The drawing under review shows one solid part. Ordinate dimensions are in mm from its lowest x, y, z. A direction names the side the tool comes from. Give positions to 0.01 mm unless a question says otherwise; leave off trailing zeros. Write each loop counter-clockwise with the first axis right and the second up, starting at its lowest first coordinate (ties: lowest second). Pieces come first, ordered by that corner, then holes. Notation, with made-up numbers: M -36,-4.75 L 11,-4.75 A28 cw 11,15.25 Z; hole C -13,16 d5. An arc over 180 degrees is marked long. Write each question's results on one line, items separated by ' | '. Start each with the question number.
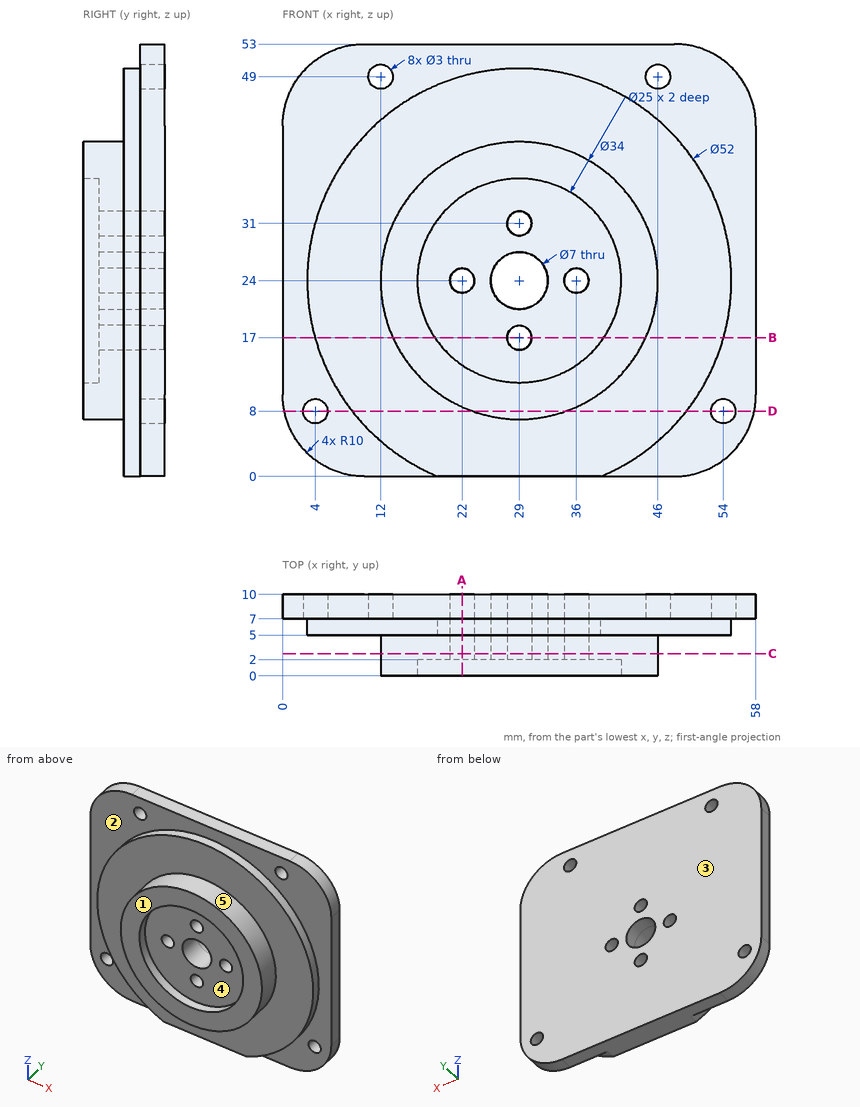
Q1. We need section B-B on z = 17. Write out the cut boundary in (x, y).
Q2. For pin 1 Ø3.5 at (x, z) = (22, 24) entering from -Y; pin 2 Ø2.5 at (x, z) = (22, 24) entering from +Y; pin 3 Ø1.5 at (y, z) = (1, 23) entering from +X; pin 4 Ø1 at (x, y) = (23.5, 1.5) entering from +Z, all flat-tipped, find the tip position at first contact; note any pin that passes through.
Q3. We need section D-D on z = 8. Write out the cut boundary in (x, y).
Q4. Wall thickness on line 1 along X through (y, z) = (5.25, 24); line 2 along X through (y, z) = (4.55, 24); line 3 along X through (y, z) = (7.8, 17): over which ranges is each line inside the solid? List them lowest first. Write a range as from..to.
Q5. We need section A-A on x = 22. Write out the cut boundary in (y, z), and give its area (3 significant figures).
Q6. For the marked faces 1 and 2, list the 3-axis set-ups (+Z, -Z, +X, -X, +Y, -Y) from which the entire face can be reached by the end or side of a thin tool; tool diameter is ignored.
Q7. We need section C-C on y = 2.75. Write out the cut boundary in (x, z), and give its area (3 significant figures).
Q8. The part is to be moulded in two halves that separate along X. For the marked faces 3, 4 and 5, say which applies: pulls with the +X half, pulls with the -X half, needs draft (parallel to the pull), parting line crosses it, or undercut.
Answer sheet:
1) outline: M 0,7 L 3.96,7 L 3.96,5 L 13.51,5 L 13.51,0 L 18.64,0 L 18.64,2 L 27.5,2 L 27.5,10 L 0,10 Z; M 30.5,2 L 39.36,2 L 39.36,0 L 44.49,0 L 44.49,5 L 54.04,5 L 54.04,7 L 58,7 L 58,10 L 30.5,10 Z
2) pin 1: y = 2 | pin 2: through | pin 3: x = 46 | pin 4: z = 40.25
3) outline: M 0.2,7 L 2.5,7 L 2.5,10 L 0.2,10 Z; M 5.5,7 L 8.51,7 L 8.51,5 L 23.26,5 L 23.26,0 L 34.74,0 L 34.74,5 L 49.49,5 L 49.49,7 L 52.5,7 L 52.5,10 L 5.5,10 Z; M 55.5,7 L 57.8,7 L 57.8,10 L 55.5,10 Z
4) line 1: 3..20.5, 23.5..25.5, 32.5..34.5, 37.5..55 | line 2: 12..20.5, 23.5..25.5, 32.5..34.5, 37.5..46 | line 3: 0..27.5, 30.5..58
5) outline: M 0,8.51 L 5,8.51 L 5,0 L 10,0 L 10,22.5 L 2,22.5 L 2,13.64 L 0,13.64 Z; M 0,34.36 L 2,34.36 L 2,25.5 L 10,25.5 L 10,53 L 7,53 L 7,49.04 L 5,49.04 L 5,39.49 L 0,39.49 Z | area: 347 mm^2
6) face 1: +Z, -Z, +X, -X, -Y | face 2: -Y
7) outline: C 29,24 d34; hole C 22,24 d3; hole C 29,24 d7; hole C 29,17 d3; hole C 29,31 d3; hole C 36,24 d3 | area: 841 mm^2
8) face 3: needs draft | face 4: undercut | face 5: parting line crosses it
